Geometry: final body of the model. Coordinates: model frame, mm. A direction names the side the tool comes from. Coordinates: 2 decimals unless noted, no trailing zeros. Write each loop counter-clockwise with the first axis right and the second up, starting at its lowest first coordinate (ties: lowest second). Pieces come first, ordered by that corner, then holes. Notation, with made-up numbers: (-10.5, 57) -> (47.5, 57) arc R18 cw to (47.5, 62) -> close; hole circle Ø5 at (4, 76). An arc over 180 degrees is marked (long way). One line per item, written item: value.
```python
from build123d import *

# Parameters (mm, degrees)
EXTRUDE_1_DEPTH     = 14
SKETCH_2_R          = 1.65
CUT_EXTRUDE_1_DEPTH = 2
SKETCH_3_R          = 1.4
CUT_EXTRUDE_2_DEPTH = 14
FILLET_1_R          = 3
SKETCH_5_R          = 0.6
CUT_EXTRUDE_3_DEPTH = 10


with BuildPart() as part:
    # 草图1 → 凸台-拉伸1 (new body)
    with BuildSketch(Plane.XY):
        Polygon((-28.25, 0), (-28.25, 19), (28.25, 19), (28.25, 0), (26.25, 0), (26.25, 16), (-26.25, 16), (-26.25, 0), align=None)
    extrude(amount=EXTRUDE_1_DEPTH)

    # 草图2 → 切除-拉伸1 (cut)
    with BuildSketch(Plane(origin=(28.25, 0, 0), x_dir=(0, 0, -1), z_dir=(1, 0, 0))):
        with Locations((-7, 5)):
            Circle(SKETCH_2_R)
    extrude(amount=-CUT_EXTRUDE_1_DEPTH, mode=Mode.SUBTRACT)

    # 草图3 → 切除-拉伸2 (cut)
    with BuildSketch(Plane(origin=(0, 19, 0), x_dir=(1, 0, 0), z_dir=(0, 1, 0))):
        with Locations((-18.98, -7)):
            Circle(SKETCH_3_R)
        with Locations((10.48, -7)):
            Circle(SKETCH_3_R)
    extrude(amount=-CUT_EXTRUDE_2_DEPTH, mode=Mode.SUBTRACT)

    # 圆角1
    fillet_1_edges = [part.edges().sort_by_distance(p)[0] for p in [
        (-27.25, 0, 0),
        (27.25, 0, 0),
        (27.25, 0, 14),
        (-27.25, 0, 14),
    ]]
    fillet(fillet_1_edges, radius=FILLET_1_R)

    # 草图5 → 切除-拉伸3 (cut)
    with BuildSketch(Plane.ZY.offset(28.25)):
        with Locations((7, 9.085)):
            Circle(SKETCH_5_R)
        with Locations((7, 13.085)):
            Circle(SKETCH_5_R)
    extrude(amount=-CUT_EXTRUDE_3_DEPTH, mode=Mode.SUBTRACT)


solid = part.part
```
(1) Section C-C (x = -18.98). Return the cut outline in (y, z), then the cut area to 3 significant figures.
Responses:
outline: (16, 0) -> (19, 0) -> (19, 5.6) -> (16, 5.6) -> close; (16, 8.4) -> (19, 8.4) -> (19, 14) -> (16, 14) -> close
area: 33.6 mm2
(2) First-contact query: pin 1 (6 mm diameter, centred on x = -10.5, y = 16.5, fed in from -Z); pin 2 (4.5 mm diameter, centred on x = -18.98, z = 7, fed in from -Y). Flat tips, straight axial feed; report the tip coordinate or a pass-through.
Responses:
pin 1: stops at z = 0
pin 2: stops at y = 16
(3) Line query: line 1 (Z direction, x = -19, y = 16.5); line 2 (X direction, y = 15.75, z = 8); line 3 (Y direction, x = 27.1, z = 7). Output: solid intervals per line, ascending. Write a range as [from, to].
Responses:
line 1: z = [0, 5.6], [8.4, 14]
line 2: x = [-28.25, -26.25], [26.25, 28.25]
line 3: y = [0, 3.35], [6.65, 19]
(4) Reachability of faces 5 (the flat face through (0, 16, 7)), 6 (the cylindrical face through (27.26, 4, 8.31)), 7 (the cylindrical face through (-27.26, 9.27, 7.57)) from +Z, -Z, +X, -X, +Y, -Y: full face, straight path, thin tool, end or side. Return the list, or none.
Responses:
face 5: +Z, -Z, -Y
face 6: +X
face 7: -X
(5) Section B-B (z = 7). Return the cut outline in (x, y) (3 decimals).
Responses:
outline: (-28.25, 0) -> (-26.25, 0) -> (-26.25, 8.485) -> (-28.25, 8.485) -> close; (-28.25, 9.685) -> (-26.25, 9.685) -> (-26.25, 12.485) -> (-28.25, 12.485) -> close; (-28.25, 13.685) -> (-26.25, 13.685) -> (-26.25, 16) -> (-20.38, 16) -> (-20.38, 19) -> (-28.25, 19) -> close; (-17.58, 16) -> (9.08, 16) -> (9.08, 19) -> (-17.58, 19) -> close; (11.88, 16) -> (26.25, 16) -> (26.25, 6.65) -> (28.25, 6.65) -> (28.25, 19) -> (11.88, 19) -> close; (26.25, 0) -> (28.25, 0) -> (28.25, 3.35) -> (26.25, 3.35) -> close
(6) Section A-A (y = 14.75). Return the cut outline in (x, z).
Responses:
outline: (-28.25, 0) -> (-26.25, 0) -> (-26.25, 14) -> (-28.25, 14) -> close; (26.25, 0) -> (28.25, 0) -> (28.25, 14) -> (26.25, 14) -> close
(7) Section D-D (y = 5). Return the cut outline in (x, z), then the cut area to 3 significant figures.
Responses:
outline: (-28.25, 0) -> (-26.25, 0) -> (-26.25, 14) -> (-28.25, 14) -> close; (26.25, 0) -> (28.25, 0) -> (28.25, 5.35) -> (26.25, 5.35) -> close; (26.25, 8.65) -> (28.25, 8.65) -> (28.25, 14) -> (26.25, 14) -> close
area: 49.4 mm2
(8) Pull-direction query (X, two-part tool) for faces 1 (the flat face through (26.25, 8, 7)), 2 (the flat face through (-26.25, 8, 7)), 3 (the flat face through (27, 0, 7)), 4 (the flat face through (28.25, 10, 7)); classes: released by +X, released by -X, zero draft, split by the parting line, or undercut.
Responses:
face 1: undercut
face 2: undercut
face 3: zero draft
face 4: released by +X
